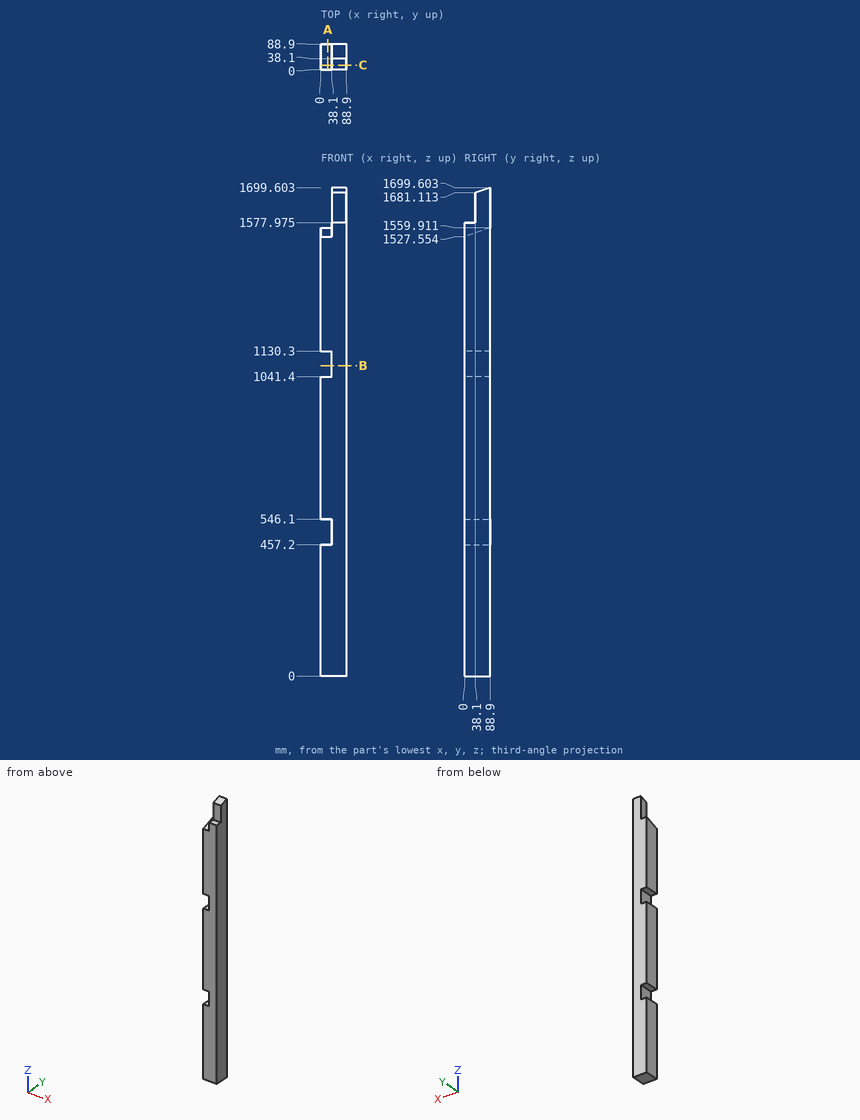
Part print with two shaded views. Sizes in mm from the minimum x, y, z corner. Round coordinates to 2 decimals unless told otherwise and drop trailing zeros. Order: outer loops, then holes, each group sorted by start corner. A loop starts at its lowest first (then second) coordinate and runs counter-clockwise, first axis right, second up. Notation, with made-up numbers: (16.5, -22.75) -> (64.5, -22.75) arc R23 ccw to (64.5, 7.25) -> close; hole circle Ø4 at (18, -15). An arc over 180 degrees is marked (long way). One line per question, with ' | ' between items.
Q1. Slice it at A-A (x = 24.5). Write the cut outline in (y, z), then the cut area to 3 significant figures.
Completed:
outline: (0, 0) -> (88.9, 0) -> (88.9, 457.2) -> (0, 457.2) -> close; (0, 546.1) -> (88.9, 546.1) -> (88.9, 1041.4) -> (0, 1041.4) -> close; (0, 1130.3) -> (88.9, 1130.3) -> (88.9, 1559.91) -> (0, 1527.55) -> close | area: 121,000 mm^2
Q2. Probe probe 1 along Z at (x, y) = (31, 81) (1 decimal); probe 2 along Z at (x, y) = (33.5, 61); probe 3 along X at (y, z) = (12.5, 1557). List the from-to ranges inside material, lowest first.
Completed:
probe 1: z = 0 to 457.2, 546.1 to 1041.4, 1130.3 to 1557 | probe 2: z = 0 to 457.2, 546.1 to 1041.4, 1130.3 to 1549.76 | probe 3: x = 38.1 to 88.9
Q3. Slice it at B-B (z = 1080). Write the cut outline in (x, y).
Completed:
outline: (38.1, 0) -> (88.9, 0) -> (88.9, 88.9) -> (38.1, 88.9) -> close
Q4. Drop flat-ended pins along their axis: pin 1 (5 mm diameter, centred on x = 41, y = 79, fed in from +Z); pin 2 (11.5 mm diameter, centred on x = 14.5, y = 61, fed in from +Z). Give the stop position or say it passes through.
Completed:
pin 1: stops at z = 1696.91 | pin 2: stops at z = 1551.85
Q5. Slice it at C-C (y = 15.5). Write the cut outline in (x, z) (1 decimal), then the cut area to 3 significant figures.
Completed:
outline: (0, 0) -> (88.9, 0) -> (88.9, 1578) -> (38.1, 1578) -> (38.1, 1533.2) -> (0, 1533.2) -> (0, 1130.3) -> (38.1, 1130.3) -> (38.1, 1041.4) -> (0, 1041.4) -> (0, 546.1) -> (38.1, 546.1) -> (38.1, 457.2) -> (0, 457.2) -> close | area: 132,000 mm^2
